from build123d import *

# Parameters (mm, degrees)
SKETCH_2_R      = 2.5
EXTRUDE_1_DEPTH = 1500


with BuildPart() as part:
    # 草图2 → 凸台-拉伸1 (new body)
    with BuildSketch(Plane.XY):
        Polygon((-18.1, 37), (-18.1, 40), (-33, 40), (-33, 2.049564589), (-30, 2.049564589), (-30, 6.348214799), (-27.5, 6.348214799), (-27.5, 3.593219783), (-24, 3.593219783), (-24, 1.376590931), (-22.4, 1.376590931), (-22.4, -1.376590931), (-24, -1.376590931), (-24, -3.593219783), (-27.5, -3.593219783), (-27.5, -6.348214799), (-30, -6.348214799), (-30, -2.049564589), (-33, -2.049564589), (-33, -9.06837916), (-30.729793093, -9.06837916), (-30.729793093, -7.473013176), (-29.144133649, -7.473013176), (-29.144133649, -9.06837916), (-27.8, -9.06837916), (-27.8, -10.56837916), (-27.8, -12.06837916), (-29.144133649, -12.06837916), (-29.144133649, -13.663745144), (-30.729793093, -13.663745144), (-30.729793093, -12.06837916), (-33, -12.06837916), (-33, -40), (-12.5, -40), (-12.5, -17), (12.5, -17), (12.5, -40), (33, -40), (33, -12.06837916), (30.729793093, -12.06837916), (30.729793093, -13.663745144), (29.144133649, -13.663745144), (29.144133649, -12.06837916), (27.8, -12.06837916), (27.8, -10.56837916), (27.8, -9.06837916), (29.144133649, -9.06837916), (29.144133649, -7.473013176), (30.729793093, -7.473013176), (30.729793093, -9.06837916), (33, -9.06837916), (33, -2.049564589), (30, -2.049564589), (30, -6.348214799), (27.5, -6.348214799), (27.5, -3.593219783), (24, -3.593219783), (24, -1.376590931), (22.4, -1.376590931), (22.4, 1.376590931), (24, 1.376590931), (24, 3.593219783), (27.5, 3.593219783), (27.5, 6.348214799), (30, 6.348214799), (30, 2.049564589), (33, 2.049564589), (33, 40), (18.1, 40), (18.1, 37), (22.1, 37), (22.1, 34.5), (20.1, 34.5), (20.1, 31), (17.5, 31), (17.5, 29.4), (12.5, 29.4), (12.5, 31), (9.9, 31), (9.9, 34.5), (7.9, 34.5), (7.9, 37), (11.9, 37), (11.9, 40), (-11.9, 40), (-11.9, 37), (-7.9, 37), (-7.9, 34.5), (-9.9, 34.5), (-9.9, 31), (-12.5, 31), (-12.5, 29.4), (-17.5, 29.4), (-17.5, 31), (-20.1, 31), (-20.1, 34.5), (-22.1, 34.5), (-22.1, 37), align=None)
        with Locations((-27.8, -33.5)):
            Circle(SKETCH_2_R, mode=Mode.SUBTRACT)
        Polygon((-20.943121928, -13.45406673), (-20.943121928, -8.11004262), (-15.8, -15.86033199), (-15.8, -31.360910729), (-24, -31.360910729), (-24, -25.86703472), (-26.644243735, -25.86703472), (-26.644243735, -13.45406673), align=None, mode=Mode.SUBTRACT)
        with Locations((27.8, -33.5)):
            Circle(SKETCH_2_R, mode=Mode.SUBTRACT)
        Polygon((24, -25.86703472), (24, -31.360910729), (15.8, -31.360910729), (15.8, -15.86033199), (20.943121928, -8.11004262), (20.943121928, -13.45406673), (26.644243735, -13.45406673), (26.644243735, -25.86703472), align=None, mode=Mode.SUBTRACT)
        with Locations((-27.8, 33.5)):
            Circle(SKETCH_2_R, mode=Mode.SUBTRACT)
        Polygon((-24.000227571, 17.552802839), (-24.000227571, 21.788095294), (-17.932238887, 21.788095294), (-17.932238887, 24.712463894), (-10.638888278, 24.712463894), (-10.638888278, 28.169211595), (-4.9, 28.169211595), (-4.9, 37), (4.9, 37), (4.9, 28.169211595), (10.638888278, 28.169211595), (10.638888278, 24.712463894), (17.932238887, 24.712463894), (17.932238887, 21.788095294), (24.000227571, 21.788095294), (24.000227571, 17.552802839), (20.143121928, 17.552802839), (20.143121928, 14.174652905), (17.932238887, 14.174652905), (17.932238887, -5.752091446), (12.045824189, -14), (0, -14), (-12.045824189, -14), (-17.932238887, -5.752091446), (-17.932238887, 14.174652905), (-20.143121928, 14.174652905), (-20.143121928, 17.552802839), align=None, mode=Mode.SUBTRACT)
        with Locations((27.8, 33.5)):
            Circle(SKETCH_2_R, mode=Mode.SUBTRACT)
    extrude(amount=EXTRUDE_1_DEPTH)


solid = part.part
The listing builds one solid part. Answer for the finished solid, in the listing's coordinates (mm). A direction names the side the tool comes from. Give positions to 0.01 mm unless a question says otherwise; leave off trailing zeros. Use one line per item in the form item = value.
1) Find section A-A on z = 225.5. Give the number of separate pieces and of enclosed holes in the cut face, and give its area (3 significant figures).
Verdict:
separate_pieces = 1
enclosed_holes = 7
area = 2,300 mm^2
2) For faces 4 (the flat face through (-33, 21, 740)), 5 (the flat face through (12.5, -28, 740)), determine the directions among +Z, -Z, +X, -X, +Y, -Y from which every point of the face is accessible in a straight line to the end or side of a thin tool.
Verdict:
face_4 = +Z, -Z, -X, +Y, -Y
face_5 = +Z, -Z, -Y
3) The mould has two halves that part along Y. Classify faces 1 (the flat face through (0, 40, 740)), 2 (the flat face through (0, -14, 740)), 3 (the flat face through (33, -26, 740)): released by +Y, released by -Y, zero draft, split by the parting line, or undercut.
Verdict:
face_1 = released by +Y
face_2 = undercut
face_3 = zero draft
4) Consider probe 1 along Y at (x, z) = (-9, 634); probe 2 along X at (y, z) = (-29.5, 482); probe 3 along X at (y, z) = (-18, 996). Determine where each line is inside the solid, lowest interval first. Write a range as [from, to].
Verdict:
probe_1 = [-17, -14], [28.17, 34.5], [37, 40]
probe_2 = [-33, -24], [-15.8, -12.5], [12.5, 15.8], [24, 33]
probe_3 = [-33, -26.64], [-15.8, -12.5], [12.5, 15.8], [26.64, 33]
